Work out the finished part from the listing and answer in its coordinate system (mm). Face numbers are marked on the shaded views. Coordinates: 2 decimals unless noted, no trailing zeros. Order: outer loops, then holes, each group sorted by start corner. A loop starts at its lowest first (then second) coordinate and runs counter-clockwise, first axis right, second up. Notation, with made-up numbers: (-16, 33) - (31, 33) arc R16 cw to (31, 64) - close; hole circle Ø4 at (-12, 9). An arc over 180 degrees is marked (long way). Answer as a JSON object with one key per item and string values. Group by question number.
1) Find the intervals of material crossed by line 1 along X through (y, z) = (9, 9.5); line 2 along X through (y, z) = (7.5, 15); line 3 along X through (y, z) = (0, 23.5), in increasing order.
2) The mould has two halves that part along Z. Classify the marked faces 1, 2 and 3: released by +Z, released by -Z, zero draft, split by the parting line, or undercut.
3) Section B-B (x = 0) is taken. Give the vertices of the cut face in (y, z).
4) Section A-A (z = 4) is taken. Count the separate pieces of the cut face and the enclosed holes in it, plus the area to 3 significant figures.
5) Each of these flat-tipped pins is pushed along its axis until it touches: P1, Ø12, axis at y = 15, z = 5.5, coming from the +X side; P2, Ø2, axis at x = -38, z = 23, coming from the -Y side; P3, Ø2, axis at y = 0.5, z = 33.5, coming from the +X side. Where does it stop, or does it pass through?
from build123d import *

# Parameters (mm, degrees)
F1_DEPTH = 15.7734
F2_DEPTH = 40.2336
F3_DEPTH = 15.7734
F4_R     = 3.302


with BuildPart() as f1:
    # F0 (on Top) → F1 (new body)
    with BuildSketch(Plane.XY):
        with BuildLine():
            ThreePointArc((3.3617647059, 18.7510276535), (-12.2241744579, 14.6106830375), (-19.05, 0))
            ThreePointArc((-19.05, 0), (-12.2241744579, -14.6106830375), (3.3617647059, -18.7510276535))
            ThreePointArc((3.3617647059, -18.7510276535), (14.6106830375, -12.2241744579), (19.05, 0))
            ThreePointArc((19.05, 0), (14.6106830375, 12.2241744579), (3.3617647059, 18.7510276535))
        make_face()
        with BuildLine():
            ThreePointArc((10.16, 0), (0, -10.16), (-10.16, 0))
            ThreePointArc((-10.16, 0), (0, 10.16), (10.16, 0))
        make_face(mode=Mode.SUBTRACT)
        with BuildLine():
            Line((-25.4, 0), (-19.05, 0))
            ThreePointArc((-19.05, 0), (-12.2241744579, 14.6106830375), (3.3617647059, 18.7510276535))
            Line((3.3617647059, 18.7510276535), (-48.9323529132, 28.1265414752))
            ThreePointArc((-48.9323529132, 28.1265414752), (-32.0589754346, 18.3362616759), (-25.4, 0))
        make_face()
    extrude(amount=F1_DEPTH)

    # F0 (on Top) → F2 (join)
    with BuildSketch(Plane.XY):
        with BuildLine():
            ThreePointArc((-48.9323529412, -28.1265414802), (-32.0589754437, -18.3362616868), (-25.4, 0))
            ThreePointArc((-25.4, 0), (-32.0589754346, 18.3362616759), (-48.9323529132, 28.1265414752))
            ThreePointArc((-48.9323529132, 28.1265414752), (-82.55, 1.42e-08), (-48.9323529412, -28.1265414802))
        make_face()
        with BuildLine():
            Line((-35.8466429449, 3.3609804232), (-35.8466429449, 0))
            Line((-35.8466429449, 0), (-35.8466429449, -3.3609804232))
            Line((-35.8466429449, -3.3609804232), (-40.0884429449, -3.3609804232))
            ThreePointArc((-40.0884429449, -3.3609804232), (-68.2625, 0), (-40.0884429449, 3.3609804232))
            Line((-40.0884429449, 3.3609804232), (-35.8466429449, 3.3609804232))
        make_face(mode=Mode.SUBTRACT)
    extrude(amount=F2_DEPTH)

    # F0 (on Top) → F3 (join)
    with BuildSketch(Plane.XY):
        with BuildLine():
            ThreePointArc((3.3617647059, -18.7510276535), (-12.2241744579, -14.6106830375), (-19.05, 0))
            Line((-19.05, 0), (-25.4, 0))
            ThreePointArc((-25.4, 0), (-32.0589754437, -18.3362616868), (-48.9323529412, -28.1265414802))
            Line((-48.9323529412, -28.1265414802), (3.3617647059, -18.7510276535))
        make_face()
    extrude(amount=F3_DEPTH)

    # F4
    f4_edges = [f1.edges().sort_by_distance(p)[0] for p in [
        (-59.017647, 28.126541, 40.2336),
    ]]
    fillet(f4_edges, radius=F4_R)


solid = f1.part
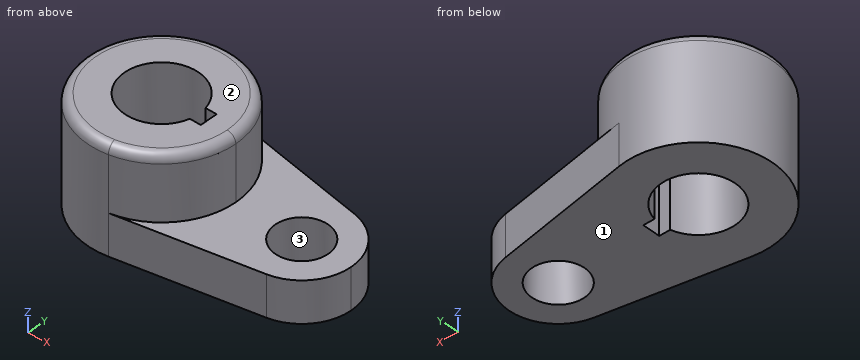
Report:
{
 "1": {"line 1": "x = -81.1 to -65.07, -42.88 to -4.71, 4.71 to 16.79", "line 2": "x = -81.55 to -66.14, -41.81 to -6.85, 6.85 to 17.51", "line 3": "x = -82.55 to -68.26, -35.85 to -25.4"},
 "2": {"face 1": "released by -Z", "face 2": "released by +Z", "face 3": "zero draft"},
 "3": {"outline": "(-19.35, 0) - (-10.16, 0) - (-10.16, 15.77) - (-19.35, 15.77) - close; (10.16, 0) - (19.35, 0) - (19.35, 15.77) - (10.16, 15.77) - close"},
 "4": {"separate pieces": "1", "enclosed holes": "2", "area": "3,470 mm²"},
 "5": {"P1": "stops at x = 16.79", "P2": "stops at y = -24.34", "P3": "stops at x = -25.4"}
}
